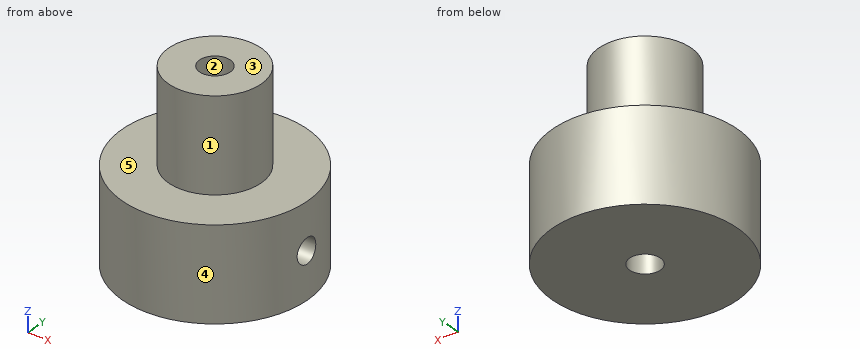
from build123d import *

# Parameters (mm, degrees)
F0_R     = 9.525
F0_R_2   = 1.5875
F1_DEPTH = 9.525
F2_R     = 4.7625
F2_R_2   = 1.5875
F3_DEPTH = 9.525
F5_R     = 1.27
F6_DEPTH = 9.525


with BuildPart() as f1:
    # F0 (on Top) → F1 (new body)
    with BuildSketch(Plane.XY):
        Circle(F0_R)
        Circle(F0_R_2, mode=Mode.SUBTRACT)
    extrude(amount=F1_DEPTH)

    # F2 (on face) → F3 (join)
    with BuildSketch(Plane.XY.offset(9.525)):
        Circle(F2_R)
        Circle(F2_R_2, mode=Mode.SUBTRACT)
    extrude(amount=F3_DEPTH)

    # F5 (on offset) → F6 (cut)
    with BuildSketch(Plane.YZ.offset(9.525)):
        with Locations((0, 4.7625)):
            Circle(F5_R)
    extrude(amount=-F6_DEPTH, mode=Mode.SUBTRACT)


solid = f1.part
CAD build for the part. Positions are in the model's coordinates, mm. Face numbers are marked on the shaded views. A direction names the side the tool comes from. Round coordinates to 2 decimals unless told otherwise and drop trailing zeros. Write each loop counter-clockwise with the first axis right and the second up, starting at its lowest first coordinate (ties: lowest second). Pieces come first, ordered by that corner, then holes. Notation, with made-up numbers: (74.5, -39) -> (123.5, -39) arc R14 ccw to (123.5, -29) -> close; hole circle Ø9 at (41.25, 75.5). An arc over 180 degrees is marked (long way). Answer as a JSON object with one key per item and string values.
(1) Pin check, flat tips, straight feed: P1, Ø4, axis at x = -4, z = 2, coming from the -Y side; P2, Ø4, axis at y = -3.5, z = 6, coming from the -X side; P3, Ø1.5, axis at x = 6.5, y = 1, coming from the +Z side (3 decimals); P4, Ø2, axis at x = 1.5, y = 0, coming from the +Z side. Stop position of each tip, or through.
Reported:
{"P1": "stops at y = -9.31", "P2": "stops at x = -9.41", "P3": "stops at z = 9.525", "P4": "stops at z = 19.05"}
(2) Which spindle directions (+Z, -Z, +X, -X, +Y, -Y) get a long thin tool onto all of the face, cutting with end or side? Do the marked faces 4 and 5. Say none if no direction does.
Reported:
{"face 4": "+Z, -Z", "face 5": "+Z"}
(3) Band-saw the part on C-C, the plane z = 11.25. List the corners of the cut face in (x, y) (1 decimal).
Reported:
{"outline": "circle Ø9.5 at (0, 0); hole circle Ø3.2 at (0, 0)"}
(4) Two-plate mould, pull along Y, no slides. Class the marked faces 1, 2 and 3: +Y half, -Y half, draft (parallel to the pull), parting line (faces both ways), or undercut.
Reported:
{"face 1": "parting line", "face 2": "undercut", "face 3": "draft"}
(5) Band-saw the part on A-A, the plane y = 0. Count the separate pieces of the cut face and the enclosed holes in it, then the cut area to 3 significant figures.
Reported:
{"separate pieces": "3", "enclosed holes": "0", "area": "192 mm^2"}
(6) Probe probe 1 along Y at (x, z) = (0, 11); probe 2 along Y at (x, z) = (0, 7) (1 decimal); probe 3 along X at (y, z) = (-8.25, 7.75). List the from-to ranges inside material, lowest first. Write a range as [from, to].
Reported:
{"probe 1": "y = [-4.76, -1.59], [1.59, 4.76]", "probe 2": "y = [-9.5, -1.6], [1.6, 9.5]", "probe 3": "x = [-4.76, 4.76]"}
